Model file for the job. Use its own axes, mm. A direction names the side the tool comes from. Round coordinates to 2 decimals unless told otherwise and drop trailing zeros. Order: outer loops, then holes, each group sorted by start corner. A loop starts at its lowest first (then second) coordinate and runs counter-clockwise, first axis right, second up. Notation, with made-up numbers: M 66.25,25.25 L 111.25,25.25 A21 cw 111.25,29.25 Z; hole C 24,70.5 d11. An arc over 180 degrees is marked long. Return JSON: item names as keys, results as strings. Group by question number.
Item 1: Slice it at D-D on x = 5.25. Write the cut outline in (y, z).
Item 2: Which spindle directions (+Z, -Z, +X, -X, +Y, -Y) get a long thin tool onto all of the face, cutting with end or side? Do faces 4 (the face through (0, -25, 22)), 5 (the face through (15, 2, 2)), 6 (the face through (15, -24, 4)). Say none if no direction does.
Item 3: Pull direction X, two halves, no side cores. Call faces 1 (the face through (15, 2, 43)), 2 (the face through (27, -24, 32)), 3 (the face through (30, -24, 22)): pulls with the +X half, pulls with the -X half, needs draft (parallel to the pull), parting line crosses it, or undercut.
Item 4: Slice it at C-C on y = -38.5. Write the cut outline in (x, z).
Item 5: Probe line 1 along Z through (x, y) = (17.75, -10); line 2 along X through (y, z) = (-46, 8); line 3 along Y through (x, z) = (3, 22). List the from-to ranges inside material, lowest first.
Item 6: Slice it at B-B on x = 12. Write the cut outline in (y, z).
Item 7: Slice it at A-A on z = 5.5. Write the cut outline in (x, y), then the cut area to 3 significant figures.
from build123d import *

# Parameters (mm, degrees)
F1_W     = 30
F1_H     = 50
F2_DEPTH = 45
F3_W     = 4
F3_H     = 2
F4_DEPTH = 1
F5_W     = 24
F5_H     = 17.5
F6_DEPTH = 53.0006863286


with BuildPart() as f2:
    # F1 (on Top) → F2 (new body)
    with BuildSketch(Plane.XY):
        Polygon((30, 2.9996863286), (0, 0), (30, 0), align=None)
        with Locations((15, -25)):
            Rectangle(F1_W, F1_H)
    extrude(amount=F2_DEPTH)

    # F3 (on face) → F4 (join)
    with BuildSketch(Plane(origin=(0, 0, 0), x_dir=(-0.9950382202, -0.0994934182, 0), z_dir=(-0.0994934182, 0.9950382202, 0))):
        with Locations((-13.0747978268, 1)):
            Rectangle(F3_W, F3_H)
        with Locations((-17.0747978268, 1)):
            Rectangle(F3_W, F3_H)
        Polygon((-11.0747978268, 45), (-15.0747978268, 45), (-19.0747978268, 45), (-19.0747978268, 43), (-15.0747978268, 43), (-11.0747978268, 43), align=None)
    extrude(amount=F4_DEPTH)

    # F5 (on face) → F6 (cut, through all)
    with BuildSketch(Plane.XZ.offset(50)):
        with Locations((15, 12.75)):
            Rectangle(F5_W, F5_H)
        with Locations((15, 32.25)):
            Rectangle(F5_W, F5_H)
    extrude(amount=-F6_DEPTH, mode=Mode.SUBTRACT)


solid = f2.part
Output values:
{
 "1": {"outline": "M -50,0 L 0.52,0 L 0.52,4 L -50,4 Z; M -50,21.5 L 0.52,21.5 L 0.52,23.5 L -50,23.5 Z; M -50,41 L 0.52,41 L 0.52,45 L -50,45 Z"},
 "2": {"face 4": "+Z, -Z, -X, +Y, -Y", "face 5": "-X, +Y", "face 6": "+Y, -Y"},
 "3": {"face 1": "needs draft", "face 2": "undercut", "face 3": "pulls with the +X half"},
 "4": {"outline": "M 0,0 L 30,0 L 30,45 L 0,45 Z; hole M 3,4 L 27,4 L 27,21.5 L 3,21.5 Z; hole M 3,23.5 L 27,23.5 L 27,41 L 3,41 Z"},
 "5": {"line 1": "0 to 4, 21.5 to 23.5, 41 to 45", "line 2": "0 to 3, 27 to 30", "line 3": "-50 to 0.3"},
 "6": {"outline": "M -50,0 L 2.2,0 L 2.2,2 L 1.2,2 L 1.2,4 L -50,4 Z; M -50,21.5 L 1.2,21.5 L 1.2,23.5 L -50,23.5 Z; M -50,41 L 1.2,41 L 1.2,43 L 2.2,43 L 2.2,45 L -50,45 Z"},
 "7": {"outline": "M 0,-50 L 3,-50 L 3,0.3 L 0,0 Z; M 27,-50 L 30,-50 L 30,3 L 27,2.7 Z", "area": "309 mm²"}
}
